```python
from build123d import *

# Parameters (mm, degrees)
SKETCH1_W           = 50
SKETCH1_H           = 100
BOSS_EXTRUDE1_DEPTH = 10
SKETCH2_R           = 4.25
SKETCH2_R_2         = 1.6
CUT_EXTRUDE2_DEPTH  = 11


with BuildPart() as part:
    # Sketch1 → Boss-Extrude1 (new body)
    with BuildSketch(Plane.XY):
        with Locations((0, 50)):
            Rectangle(SKETCH1_W, SKETCH1_H)
    extrude(amount=BOSS_EXTRUDE1_DEPTH)

    # Sketch2 → Cut-Extrude2 (cut)
    with BuildSketch(Plane.XY):
        with Locations(Location((0, 75, 0), (0, 0, 180))):
            Circle(SKETCH2_R)
        with Locations(Location((15, 6, 0), (0, 0, 180))):
            Circle(SKETCH2_R_2)
        with Locations(Location((-15, 6, 0), (0, 0, 180))):
            Circle(SKETCH2_R_2)
    extrude(amount=CUT_EXTRUDE2_DEPTH, mode=Mode.SUBTRACT)


solid = part.part
```
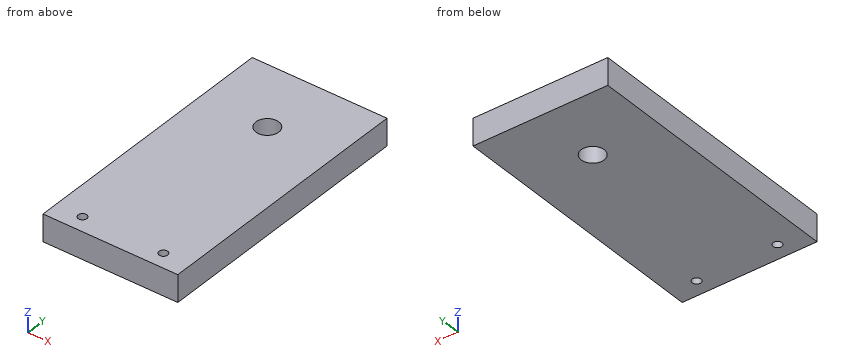
Verification items for the finished model (mm, model axes). Coordinates: 2 decimals unless noted, no trailing zeros. Write each loop counter-clockwise with the first axis right and the second up, starting at its lowest first coordinate (ties: lowest second). Pieces come first, ordered by that corner, then holes. Notation, with made-up numbers: (47.25, -7.5) - (95.25, -7.5) arc R30 cw to (95.25, 24.5) - close; hole circle Ø3 at (-8.5, -21.5). An arc over 180 degrees is marked (long way). One line per question, with ' | ' between items. Start each with the question number.
1. Material ranges on line 1 along X through (y, z) = (6, 5); line 2 along Y through (x, z) = (-15, 3); line 3 along Y through (x, z) = (0, 5.5), recorded low to high.
2. Section check B-B (y = 75). Enter the section's corners in (x, z), plus the area to 3 significant figures.
3. Section check A-A (x = 0). Enter the section's corners in (y, z), plus the area to 3 significant figures.
Computed values:
1) line 1: -25 to -16.6, -13.4 to 13.4, 16.6 to 25 | line 2: 0 to 4.4, 7.6 to 100 | line 3: 0 to 70.75, 79.25 to 100
2) outline: (-25, 0) - (-4.25, 0) - (-4.25, 10) - (-25, 10) - close; (4.25, 0) - (25, 0) - (25, 10) - (4.25, 10) - close | area: 415 mm²
3) outline: (0, 0) - (70.75, 0) - (70.75, 10) - (0, 10) - close; (79.25, 0) - (100, 0) - (100, 10) - (79.25, 10) - close | area: 915 mm²
